Check sheet for the drawn part. Datum: minimum x, y, z corner. Units: mm. Coordinates: 2 decimals unless noted, no trailing zeros. Write each loop counter-clockwise with the first axis right and the second up, starting at its lowest first coordinate (ties: lowest second). Pieces come first, ordered by that corner, then holes. Notation, with made-up numbers: (47.5, 34) -> (71.5, 34) arc R28 ccw to (71.5, 64) -> close; hole circle Ø7 at (-39, 78.25). An arc over 180 degrees is marked (long way). Answer in a Markdown table with one row per item. Add a question column.
1. Cross-section at D-D on z = 0.75. Record the cut outline in (x, y), and give its area (3 significant figures).
2. Cross-section at C-C on x = 21. Record the cut outline in (y, z), and give its area (3 significant figures).
3. Cross-section at B-B on y = 0.3. Record the cut outline in (x, z) (3 decimals), and give its area (3 significant figures).
4. Cross-section at A-A on z = 4.1. Record the cut outline in (x, y) (3 decimals), and give its area (3 significant figures).
5. Scan lines: L1, parallel to X at y = 0.35, z = 4.1 (3 decimals); L2, parallel to X at y = 0.3, z = 4; L3, parallel to Z at x = 22.5, y = 0.25. Record each from-to range of solid material in increasing order. Write a range as from..to.
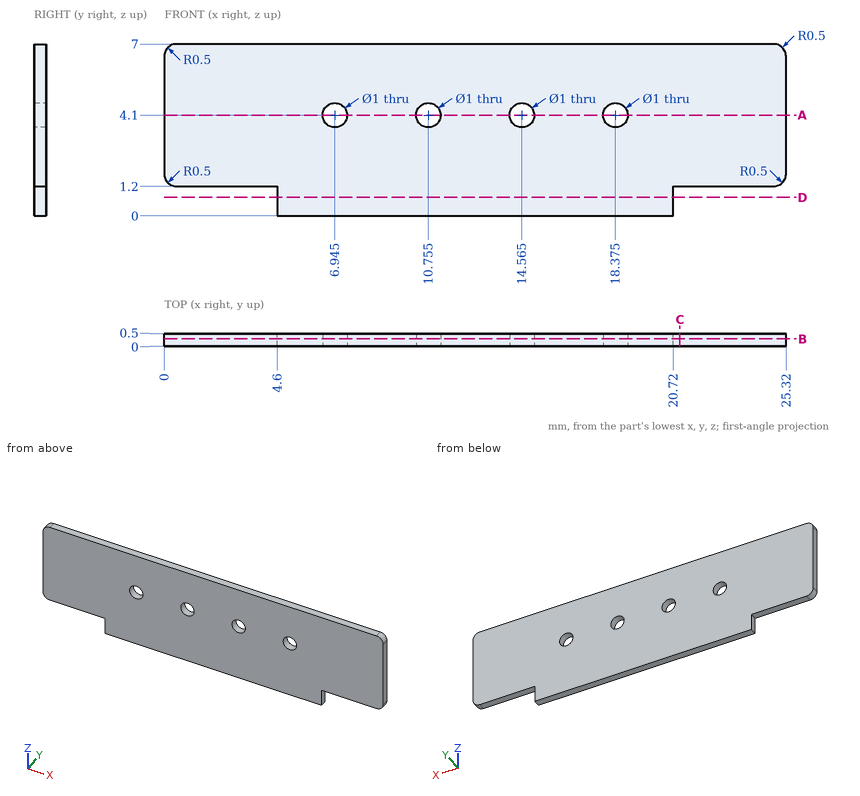
Results found:
| question | item | result |
|---|---|---|
| 1 | outline | (4.6, 0) -> (20.72, 0) -> (20.72, 0.5) -> (4.6, 0.5) -> close |
| 1 | area | 8.06 mm^2 |
| 2 | outline | (0, 1.2) -> (0.5, 1.2) -> (0.5, 7) -> (0, 7) -> close |
| 2 | area | 2.90 mm^2 |
| 3 | outline | (0, 1.7) arc R0.5 ccw to (0.5, 1.2) -> (4.6, 1.2) -> (4.6, 0) -> (20.72, 0) -> (20.72, 1.2) -> (24.82, 1.2) arc R0.5 ccw to (25.32, 1.7) -> (25.32, 6.5) arc R0.5 ccw to (24.82, 7) -> (0.5, 7) arc R0.5 ccw to (0, 6.5) -> close; hole circle Ø1 at (6.945, 4.1); hole circle Ø1 at (10.755, 4.1); hole circle Ø1 at (14.565, 4.1); hole circle Ø1 at (18.375, 4.1) |
| 3 | area | 163 mm^2 |
| 4 | outline | (0, 0) -> (6.445, 0) -> (6.445, 0.5) -> (0, 0.5) -> close; (7.445, 0) -> (10.255, 0) -> (10.255, 0.5) -> (7.445, 0.5) -> close; (11.255, 0) -> (14.065, 0) -> (14.065, 0.5) -> (11.255, 0.5) -> close; (15.065, 0) -> (17.875, 0) -> (17.875, 0.5) -> (15.065, 0.5) -> close; (18.875, 0) -> (25.32, 0) -> (25.32, 0.5) -> (18.875, 0.5) -> close |
| 4 | area | 10.7 mm^2 |
| 5 | L1 | x = 0..6.445, 7.445..10.255, 11.255..14.065, 15.065..17.875, 18.875..25.32 |
| 5 | L2 | x = 0..6.46, 7.43..10.27, 11.24..14.08, 15.05..17.89, 18.86..25.32 |
| 5 | L3 | z = 1.2..7 |
